Autodesk Inventor part; units mm, degrees
ref_plane "Work Plane1" through (104.775, 0, 0) normal (0, 0, -1) x (1, 0, 0)
ref_plane "YZ Plane" through (0, 0, 0) normal (1, 0, 0) x (0, 1, 0)
ref_plane "XZ Plane" through (0, 0, 0) normal (0, 1, 0) x (-1, 0, 0)
sketch "Esquisse1" plane through (0, 0, 0) normal (0, 0, 1) x (1, 0, 0)
  line L0 (12, 0) -> (12, 2.5)
  line L1 (12, 2.5) -> (5.6, 2.5)
  line L2 (5.6, 2.5) -> (5.1092, 2.5)
  line L3 (0, 4.715) -> (0, 1.7321)
  line L4 (0, 1.7321) -> (2.14, 1.7321)
  line L5 (2.14, 1.7321) -> (3.14, 0)
  line L6 (3.14, 0) -> (12, 0)
  line L7 (0, 4.715) -> (0.885, 4.715)
  line L8 (0.885, 4.715) -> (3.1, 2.5)
  line L9 (5.1092, 2.5) -> (3.1, 2.5)
  line L10 (5.6, 2.5) -> (3.1, 2.5) construction
  line L11 (3.1, 2.5) -> (3.1, 2.5)
  line L12 (-2.4, 0) -> (14.4, 0)
  line L13 (0, -0.943) -> (0, 5.658)
  dimension "d0" = 12
  dimension "d1" = 6.4
  dimension "d2" = 2.14
  dimension "d3" = 5
  dimension "d6" = 3.1
  dimension "d7" = 45
  dimension "d8" = 3.4641
  dimension "d9" = 60
  dimension "d10" = 9.43
  dimension "d11" = 5
  dimension "d12" = 0.4908
revolve "Corps" add sketch "Esquisse1" angle 360 about axis through (3.14, 0, 0) along (1, 0, 0) contours L6 L5 L4 L3 L7 L8 L9 L2 L1 L0
sketch "Esquisse2" plane through (0, 0, 0) normal (-1, 0, 0) x (0, 0, 1)
  circle A0 centre (0, 0) radius 1.7321
  line L0 (0, -6.601) -> (0, 6.601)
  line L1 (-6.601, 0) -> (6.601, 0)
  line L2 (1.7321, 0) -> (0.866, -1.5)
  line L3 (0.866, -1.5) -> (-0.866, -1.5)
  line L4 (-0.866, -1.5) -> (-1.7321, 0)
  line L5 (-1.7321, 0) -> (-0.866, 1.5)
  line L6 (-0.866, 1.5) -> (0.866, 1.5)
  line L7 (0.866, 1.5) -> (1.7321, 0)
  point P0 (0, 1.7321)
extrude "Rainure" add sketch "Esquisse2" against normal up to next contours L7 A0 | A0 L2 | L6 L0 A0 | A0 L0 L3 | L0 L6 A0 | A0 L3 L0 | L4 A0 | A0 L5
thread "Filetage"
chamfer "Chanfrein1" distance 0.4908 distance2 0.4908 1 edges at (12, -2.5, 0) measured on face at (12, -0.6238, 0.9515)
ref_plane "Work Plane1" through (104.775, 0, 0) normal (0, 0, -1) x (1, 0, 0)
equation "\"d15\" = GEL"
equation "\"d17\" = -0.5 * SPD + 0.5 * GD"
equation "\"d18\" = GUL"
equation "\"d0\" = NLG"
equation "\"d1\" = GEL"
equation "\"d2\" = INTI"
equation "\"d3\" = GD"
equation "\"d6\" = KOH"
equation "\"d7\" = 0.5 * SEWI"
equation "\"d8\" = 1.1547 * SW"
equation "\"d10\" = KOD"
equation "\"d11\" = BDM"
equation "\"d12\" = GAL"
equation "\"NLG\" = 12"
equation "\"INTI\" = 2.14"
equation "\"GEL\" = 6.4"
equation "\"GAL\" = 0.61345 * PTC"
equation "\"KOH\" = 3.1"
equation "\"KOD\" = 9.43"
equation "\"GUL\" = 0.61345 * PTC"
equation "\"SPD\" = NND - 1.2269 * PTC"
equation "\"BDM\" = NND"
equation "\"GD\" = NND"
equation "\"SEWI\" = 90deg"
equation "\"SW\" = 3"
equation "\"TOA\" = 30deg"
equation "\"GD1\" = THREADDIA - 1.2269 * PTC"
equation "\"EPV\" = 5.6"
equation "\"THREADDIA\" = 5"
equation "\"PTC\" = 0.8"
equation "\"NND\" = 5"
equation "\"E0\" = 3.47"
equation "\"THREADDESC\" = 1.2345"
properties part number "ISO 10642 - M5 x  12" material "Acier"
Build history of the part. All positions in model axes, mm. A direction names the side the tool comes from. Give positions to 0.01 mm unless a question says otherwise; leave off trailing zeros. Loops run counter-clockwise (first coordinate to the right, second up) from the corner with the lowest first, then second, coordinate; pieces in that order, holes last. Notation, with made-up numbers: (35.25, 41.5) -> (58.25, 41.5) arc R27 ccw to (58.25, 69.5) -> close; hole circle Ø10 at (26, 57). An arc over 180 degrees is marked (long way). One line per question, with ' | ' between items. Start each with the question number.
1) Cut at A-A (x = 10.75). Give the cut face in (y, z).
2) Two-plate mould, pull along Y, no slides. Class faces 4 (the flat face through (1.121, 0.74, -1.305)), 5 (the flat face through (0, 0, 2)), 6 (the conical face through (2.96, -2.09, 1.61)): released by +Y, released by -Y, zero draft, split by the parting line, or undercut.
3) 3-axis set-ups, long thin cutter, end or side, ignore diameter. For faces 1 (the cylindrical face through (0.449, -0.614, 4.675)), 2 (the cylindrical face through (7.25, -0.54, 2.44)), 3 (the flat face through (1.121, 0.761, 1.293)): which of +Z, -Z, +X, -X, +Y, -Y reach the whole face in a straight line?
4) Pin check, flat tips, straight feed: pin 1 (1.5 mm diameter, centred on x = 2.5, z = 3, fed in from -Y); pin 2 (5 mm diameter, centred on x = 3, z = -2.5, fed in from -Y); pin 3 (5 mm diameter, centred on x = 3.5, y = 3, fed in from +Z). Stop position of each tip, or through.
5) Probe L1, parallel to Z at x = 1, y = 1; L2, parallel to Y at x = 4.25, z = 2; L3, parallel to Z at x = 5.5, y = 0. List the from-to ranges inside material, lowest first.
Return value:
1) outline: circle Ø5 at (0, 0)
2) face 4: undercut | face 5: zero draft | face 6: split by the parting line
3) face 1: +X, -X | face 2: +X | face 3: -X
4) pin 1: y = -2.68 | pin 2: y = -4.57 | pin 3: z = 3.91
5) L1: -4.49 to -1.15, 1.15 to 4.49 | L2: -1.5 to 1.5 | L3: -2.5 to 2.5
